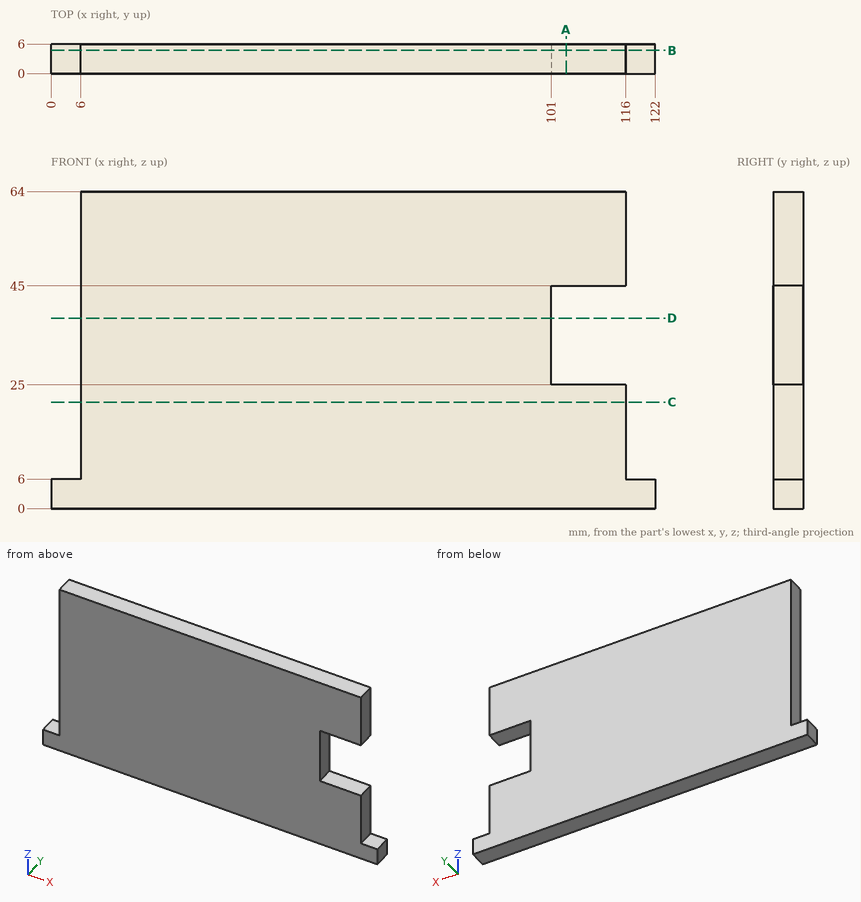
Design review of the part shown in the three views and the two pictorial views. Dimensions are in mm from the part's minimum x, y and z. Round coordinates to 2 decimals unless told otherwise and drop trailing zeros. Write each loop counter-clockwise with the first axis right and the second up, starting at its lowest first coordinate (ties: lowest second). Pieces come first, ordered by that corner, then holes.
1) For line 1 along Z through (x, y) = (115.5, 0.7); line 2 along X through (y, z) = (4.15, 9); line 3 along X through (y, z) = (4.6, 35), list the stretches that pass through material, from the lowest coordinate up.
Answer below:
line 1: z = 0 to 25, 45 to 64
line 2: x = 6 to 116
line 3: x = 6 to 101
2) Take a section at D-D on z = 38.5. Give the boundary of the cut face in (x, y).
Answer below:
outline: (6, 0) - (101, 0) - (101, 6) - (6, 6) - close
3) Take a section at A-A on x = 104. Give the boundary of the cut face in (y, z).
Answer below:
outline: (0, 0) - (6, 0) - (6, 25) - (0, 25) - close; (0, 45) - (6, 45) - (6, 64) - (0, 64) - close
4) Take a section at C-C on z = 21.5. Give the boundary of the cut face in (x, y), then the cut area to 3 significant figures.
Answer below:
outline: (6, 0) - (116, 0) - (116, 6) - (6, 6) - close
area: 660 mm2
5) Insertion check: pin 1 Ø1.5 at (y, z) = (4, 41) entering from -X; pin 2 Ø1.8 at (y, z) = (3.5, 52.5) entering from +X. Each pin has a flat end and moves straight along its axis. Give the tip position at first contact, or say it passes through.
Answer below:
pin 1: stops at x = 6
pin 2: stops at x = 116
6) Take a section at B-B on y = 4.7. Give the boundary of the cut face in (x, z).
Answer below:
outline: (0, 0) - (122, 0) - (122, 6) - (116, 6) - (116, 25) - (101, 25) - (101, 45) - (116, 45) - (116, 64) - (6, 64) - (6, 6) - (0, 6) - close
